from build123d import *

# Parameters (mm, degrees)
F2_R      = 87
F4_R      = 5
F5_DEPTH  = 93.001
F6_R      = 2.5
F7_DEPTH  = 12.5
F8_R      = 2.5
F9_DEPTH  = 12.5
F10_R     = 2.5
F11_DEPTH = 12.5


# Not quite as in the source:
# - an extrude whose draft closes it to a point is written as a loft to that point


with BuildPart() as f1:
    # F0 (on Front) → F1 (revolve)
    with BuildSketch(Plane.XZ):
        Polygon((-100, 0), (0, 0), (0, 93), (-90, 3), (-100, 3), align=None)
    revolve(axis=Axis((0, 0, 46.5), (0, 0, -1)))

    # F2 (on face) → F3 section 0
    with BuildSketch(Plane(origin=(0, 0, 0), x_dir=(1, 0, 0), z_dir=(0, 0, -1)), mode=Mode.PRIVATE) as f3_s0:
        Circle(F2_R)
    loft([f3_s0.sketch, Vertex(0, 0, 87)], ruled=True, mode=Mode.SUBTRACT)

    # F4 (on Top) → F5 (cut, through all)
    with BuildSketch(Plane.XY):
        Circle(F4_R)
    extrude(amount=F5_DEPTH, mode=Mode.SUBTRACT)

    # F6 (on face) → F7 (cut, symmetric)
    with BuildSketch(Plane.XY.offset(3)):
        with Locations((0, 94)):
            Circle(F6_R)
    extrude(amount=F7_DEPTH, both=True, mode=Mode.SUBTRACT)

    # F8 (on face) → F9 (cut, symmetric)
    with BuildSketch(Plane(origin=(0, 0, 0), x_dir=(1, 0, 0), z_dir=(0, 0, -1))):
        with Locations((-78.3080390386, 51.9985674988)):
            Circle(F8_R)
    extrude(amount=F9_DEPTH, both=True, mode=Mode.SUBTRACT)

    # F10 (on face) → F11 (cut, symmetric)
    with BuildSketch(Plane(origin=(0, 0, 0), x_dir=(1, 0, 0), z_dir=(0, 0, -1))):
        with Locations((77.6980827138, 52.9056513294)):
            Circle(F10_R)
    extrude(amount=F11_DEPTH, both=True, mode=Mode.SUBTRACT)


solid = f1.part
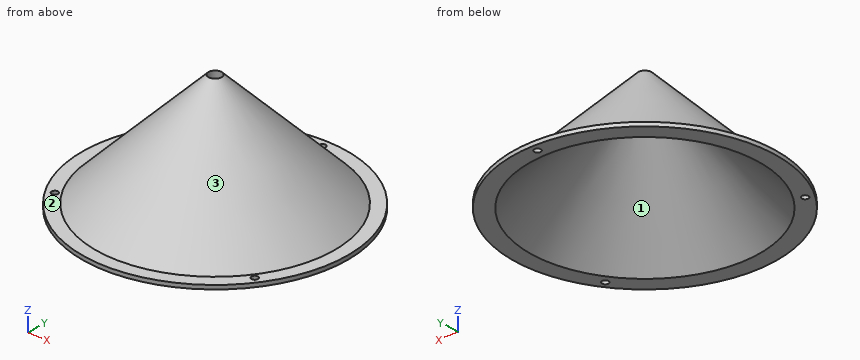
Here's how the part is built. I have some questions about the finished solid (model axes, mm). Face numbers are marked on the shaded views. Coordinates: 2 decimals unless noted, no trailing zeros. Loops run counter-clockwise (first coordinate to the right, second up) from the corner with the lowest first, then second, coordinate; pieces in that order, holes last.
1. Imagine slicing it at C-C, the plane y = 94. Please give me the cut outline in (x, z), and give its area (3 significant figures).
2. Imagine slicing it at A-A, the plane x = 0. Please give me the cut outline in (y, z), and give its area (3 significant figures).
3. Imagine slicing it at D-D, the plane z = 40.5. Please give me the cut outline in (x, y), and give its area (3 significant figures).
4. I need wall thicknesses on L1, parallel to Y at x = 0, z = 1.2; L2, parallel to Y at x = 0, z = 1.3; L3, parallel to Z at x = 19.5, y = -90.5. Which ranges of each line are inside material? Lowest first, please.
5. For P1, Ø8, axis at x = -60.5, y = -39, coming from the -Z side; P2, Ø5, axis at x = -20, z = 71, coming from the +Y side; P3, Ø8, axis at y = 47, z = 9, coming from the +X side, each with a flat end and sliding along its axis, tell me the tip position at first contact or that it passes through.
6. If we mould it in two halves opening along X, with no side actions, what happens to the marked faces 1, 2 and 3? For each: pulls with the +X half, pulls with the -X half, needs draft (parallel to the pull), parting line crosses it, or undercut.
7. Imagine slicing it at B-B, the plane z = 30. Please give me the cut outline in (x, y).
Taken from the geometry:
1. outline: (-34.12, 0) - (-2.5, 0) - (-2.5, 3) - (-34.12, 3) - close; (2.5, 0) - (34.12, 0) - (34.12, 3) - (2.5, 3) - close
1. area: 190 mm2
2. outline: (-100, 0) - (-87, 0) - (-5, 82) - (-5, 88) - (-90, 3) - (-100, 3) - close; (5, 82) - (87, 0) - (91.5, 0) - (91.5, 3) - (90, 3) - (5, 88) - close; (96.5, 0) - (100, 0) - (100, 3) - (96.5, 3) - close
2. area: 1,060 mm2
3. outline: circle Ø105 at (0, 0); hole circle Ø93 at (0, 0)
3. area: 1,870 mm2
4. L1: y = -100 to -85.8, 85.8 to 91.5, 96.5 to 100
4. L2: y = -100 to -85.7, 85.7 to 91.5, 96.5 to 100
4. L3: z = 0 to 3
5. P1: stops at z = 11.02
5. P2: stops at y = 15.29
5. P3: stops at x = 75.01
6. face 1: undercut
6. face 2: needs draft
6. face 3: parting line crosses it
7. outline: circle Ø126 at (0, 0); hole circle Ø114 at (0, 0)
